Build history of the part. All positions in model axes, mm. A direction names the side the tool comes from. Round coordinates to 2 decimals unless told otherwise and drop trailing zeros. Write each loop counter-clockwise with the first axis right and the second up, starting at its lowest first coordinate (ties: lowest second). Pieces come first, ordered by that corner, then holes. Notation, with made-up numbers: M 50.5,81 L 68.5,81 A12 ccw 68.5,93 Z; hole C 47.25,1 d5. An arc over 180 degrees is marked long. Write item = value, one per line. Start each with the question number.
Q1. Probe L1, parallel to X at y = 5.75, z = 0.6; L2, parallel to Z at x = 2.5, y = 2.35; L3, parallel to X at y = 4.35, z = 0.3. List the from-to ranges inside material, lowest first.
Q2. Tool access for faces 1 (the flat face through (0.4, 3, 2)), 2 (the flat face through (4.9, 1.7, 0)): list every direction of +Z, -Z, +X, -X, +Y, -Y with a clear straight run to the whole face (end or side of a thin tool).
Q3. Band-saw the part on D-D on y = 3.1. Write the cut outline in (x, z), plus the area to 3 significant figures.
Q4. Band-saw the part on B-B on z = 3.85. Write the cut outline in (x, y).
Q5. Band-saw the part on A-A on y = 1.15. Write the cut outline in (x, z).
Q6. Band-saw the part on C-C on x = 8.75. Write the cut outline in (y, z), plus the area to 3 significant figures.
Q7. Drop a flat-ended pin along its axis: P1, Ø2, axis at x = 4.5, z = 2.5, coming from the +Y side. Give the stop position or say it passes through.
Q8. Pull direction X, two halves, no side cores. Call faces 3 (the flat face through (5, 0, 2)), 4 (the flat face through (5, 1, 0.4)), 5 (the flat face through (0, 3, 2)): released by +X, released by -X, zero draft, split by the parting line, or undercut.
```python
from build123d import *

# Parameters (mm, degrees)
SKETCH_1_W          = 10
SKETCH_1_H          = 6
EXTRUDE_1_DEPTH     = 5
SHELL_1_T           = -0.4
CUT_EXTRUDE_1_REACH = 14.689
SKETCH_2_W          = 4
SKETCH_2_H          = 4


with BuildPart() as part:
    # 草图1 → 凸台-拉伸1 (new body)
    with BuildSketch(Plane.XY):
        with Locations((5, 3)):
            Rectangle(SKETCH_1_W, SKETCH_1_H)
    extrude(amount=EXTRUDE_1_DEPTH)

    # 抽壳1
    shell_1_openings = [part.faces().sort_by_distance(p)[0] for p in [
        (5, 6, 2.5),
    ]]
    offset(amount=SHELL_1_T, openings=shell_1_openings, kind=Kind.INTERSECTION)

    # 草图2 → 切除-拉伸1 (cut, up to next)
    with BuildSketch(Plane(origin=(0, 0, 0), x_dir=(-1, 0, 0), z_dir=(0, 0, -1)), mode=Mode.PRIVATE) as cut_extrude_1_sk1:
        with Locations((-5, 4)):
            Rectangle(SKETCH_2_W, SKETCH_2_H)
    cut_extrude_1_tool1 = extrude(cut_extrude_1_sk1.sketch, amount=-CUT_EXTRUDE_1_REACH, mode=Mode.PRIVATE) & part.part
    add(cut_extrude_1_tool1.solids().sort_by_distance((5, 4, 0))[0], mode=Mode.SUBTRACT)


solid = part.part
```
Conclusion:
q1.L1 = 0 to 0.4, 9.6 to 10
q1.L2 = 0 to 0.4, 4.6 to 5
q1.L3 = 0 to 3, 7 to 10
q2.face_1 = +Y
q2.face_2 = -Z, +X, -X, +Y, -Y
q3.outline = M 0,0 L 3,0 L 3,0.4 L 0.4,0.4 L 0.4,4.6 L 9.6,4.6 L 9.6,0.4 L 7,0.4 L 7,0 L 10,0 L 10,5 L 0,5 Z
q3.area = 9.76 mm^2
q4.outline = M 0,0 L 10,0 L 10,6 L 9.6,6 L 9.6,0.4 L 0.4,0.4 L 0.4,6 L 0,6 Z
q5.outline = M 0,0 L 10,0 L 10,5 L 0,5 Z; hole M 0.4,0.4 L 9.6,0.4 L 9.6,4.6 L 0.4,4.6 Z
q6.outline = M 0,0 L 6,0 L 6,0.4 L 0.4,0.4 L 0.4,4.6 L 6,4.6 L 6,5 L 0,5 Z
q6.area = 6.48 mm^2
q7.P1 = 0.4
q8.face_3 = zero draft
q8.face_4 = undercut
q8.face_5 = released by -X
